Study the drawing (mm; zero at the part's minimum x, y, z) and answer. A direction names the side the tool comes from. Give positions to 0.01 mm unless a question says otherwise; leave off trailing zeros. Write each loop counter-clockwise with the first axis right and the second up, starting at its lowest first coordinate (ties: lowest second). Pieces come first, ordered by that corner, then holes. Notation, with made-up numbers: (50, -33) - (58, -33) arc R16 ccw to (58, -20) - close; hole circle Ø5 at (39.5, 83.25). An arc over 180 degrees is marked (long way). Return JSON: item names as keys, results as strings.
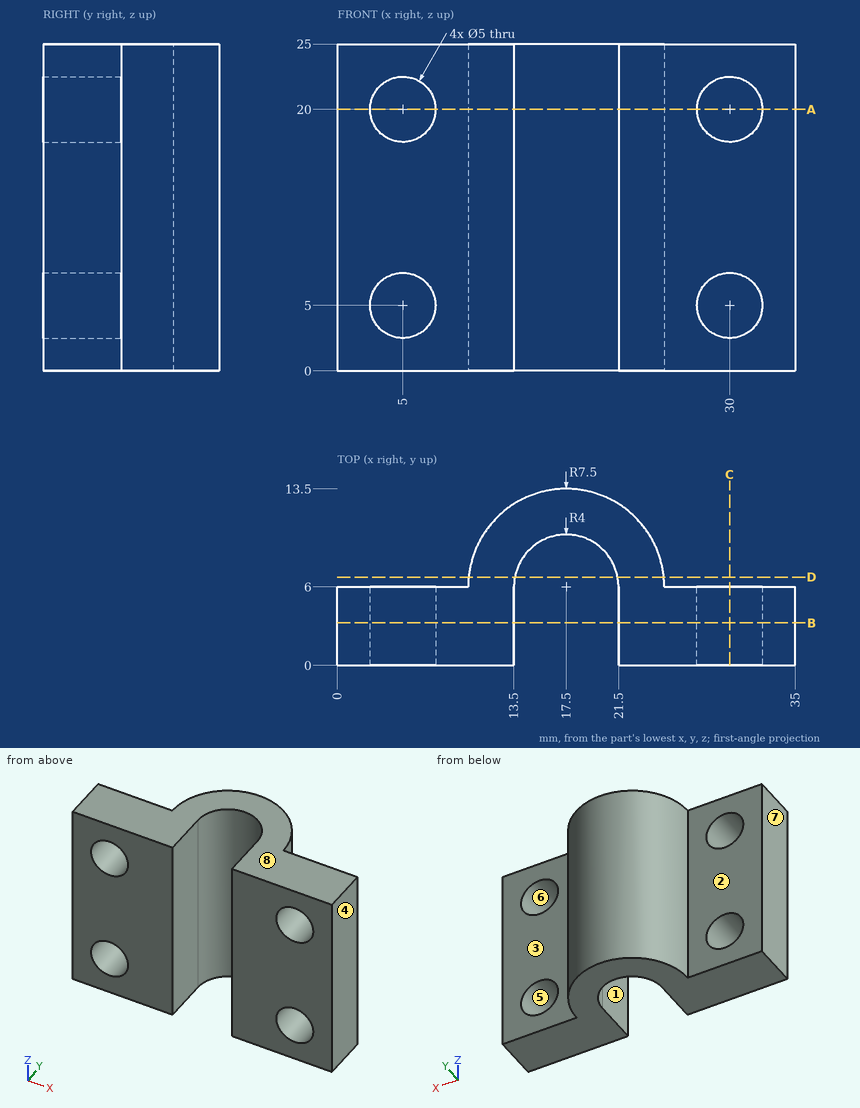
Item 1: For the marked faces 1, 2, 3 and 4, determine the directions among +Z, -Z, +X, -X, +Y, -Y from which every point of the face is accessible in a straight line to the end or side of a thin tool.
Answer below:
{"face 1": "+Z, -Z, -Y", "face 2": "+Z, -Z, -X, +Y", "face 3": "+Z, -Z, +X, +Y", "face 4": "+Z, -Z, +X, +Y, -Y"}
Item 2: A cutting plane is placed at B-B on y = 3.25. Determine the outline of the cut face in (x, z).
Answer below:
{"outline": "(0, 0) - (13.5, 0) - (13.5, 25) - (0, 25) - close; (21.5, 0) - (35, 0) - (35, 25) - (21.5, 25) - close; hole circle Ø5 at (5, 5); hole circle Ø5 at (5, 20); hole circle Ø5 at (30, 5); hole circle Ø5 at (30, 20)"}
Item 3: A cutting plane is placed at A-A on z = 20. Determine the outline of the cut face in (x, y).
Answer below:
{"outline": "(0, 0) - (2.5, 0) - (2.5, 6) - (0, 6) - close; (7.5, 0) - (13.5, 0) - (13.5, 6) arc R4 cw to (21.5, 6) - (21.5, 0) - (27.5, 0) - (27.5, 6) - (25, 6) arc R7.5 ccw to (10, 6) - (7.5, 6) - close; (32.5, 0) - (35, 0) - (35, 6) - (32.5, 6) - close"}
Item 4: Flat-ended cylindrical pins translate along their axes: P1, Ø8, axis at x = 30, z = 5, coming from the +Y side; P2, Ø5, axis at y = 11, z = 12.5, coming from the -X side; P3, Ø4, axis at x = 11.5, z = 3.5, coming from the +Y side. Find the tip coordinate at first contact, or state that the pin passes through.
Answer below:
{"P1": "stops at y = 6", "P2": "stops at x = 10.43", "P3": "stops at y = 12.34"}
Item 5: Consider L1, parallel to X at y = 3.35, z = 20; L2, parallel to Z at x = 5, y = 4.45; L3, parallel to Z at x = 4, y = 4.25. Determine where each line is inside the solid, lowest interval first.
Answer below:
{"L1": "x = 0 to 2.5, 7.5 to 13.5, 21.5 to 27.5, 32.5 to 35", "L2": "z = 0 to 2.5, 7.5 to 17.5, 22.5 to 25", "L3": "z = 0 to 2.71, 7.29 to 17.71, 22.29 to 25"}
Item 6: A cutting plane is placed at C-C on x = 30. Determine the outline of the cut face in (y, z), then the cut area to 3 significant figures.
Answer below:
{"outline": "(0, 0) - (6, 0) - (6, 2.5) - (0, 2.5) - close; (0, 7.5) - (6, 7.5) - (6, 17.5) - (0, 17.5) - close; (0, 22.5) - (6, 22.5) - (6, 25) - (0, 25) - close", "area": "90.0 mm²"}
Item 7: A cutting plane is placed at D-D on y = 6.75. Determine the outline of the cut face in (x, z).
Answer below:
{"outline": "(10.04, 0) - (13.57, 0) - (13.57, 25) - (10.04, 25) - close; (21.43, 0) - (24.96, 0) - (24.96, 25) - (21.43, 25) - close"}
Item 8: The mould has two halves that part along X. Classify the marked faces 5, 6, 7 and 8: +X half, -X half, draft (parallel to the pull), parting line (faces both ways), or undercut.
Answer below:
{"face 5": "undercut", "face 6": "undercut", "face 7": "-X half", "face 8": "draft"}
